Answer from the drawing. Dimensions are ordinates in mm from the lowest x, y and z of the part. Give positions to 0.01 mm unless a question says otherwise; leave off trailing zeros. Loops run counter-clockwise (first coordinate to the right, second up) from the corner with the lowest first, then second, coordinate; pieces in that order, holes last.
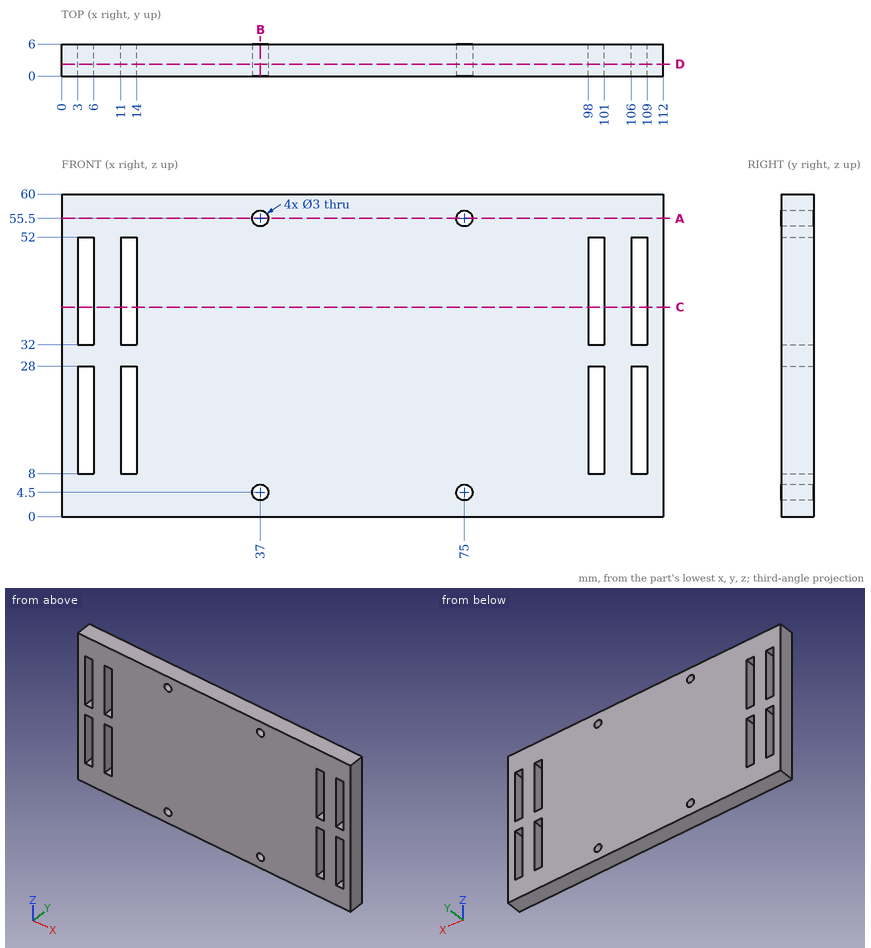
Item 1: Consider line 1 (X direction, y = 2.55, z = 4.5); line 2 (X direction, y = 5.7, z = 18); line 3 (Z direction, x = 75, y = 1.25). Determine where each line is inside the solid, lowest interval first.
Item 2: Find section B-B, the plane x = 37. Write down the section's boundary in (y, z).
Item 3: Find section C-C, the plane z = 39. Write down the section's boundary in (x, y), plus the area to 3 significant figures.
Item 4: Find section A-A, the plane z = 55.5. Write down the section's boundary in (x, y), plus the area to 3 significant figures.
Item 5: A flat-ended cylindrical pin translates along its axis: pin 1 Ø1.8 at (y, z) = (2.5, 18.5) entering from -X. Find the tip coordinate at first contact, or state that the pin passes through.
Item 6: Find section D-D, the plane y = 2.25. Give the number of separate pieces and of enclosed holes in the cut face, plus the area to 3 significant figures.
Ans:
1. line 1: x = 0 to 35.5, 38.5 to 73.5, 76.5 to 112
1. line 2: x = 0 to 3, 6 to 11, 14 to 98, 101 to 106, 109 to 112
1. line 3: z = 0 to 3, 6 to 54, 57 to 60
2. outline: (0, 0) - (6, 0) - (6, 3) - (0, 3) - close; (0, 6) - (6, 6) - (6, 54) - (0, 54) - close; (0, 57) - (6, 57) - (6, 60) - (0, 60) - close
3. outline: (0, 0) - (3, 0) - (3, 6) - (0, 6) - close; (6, 0) - (11, 0) - (11, 6) - (6, 6) - close; (14, 0) - (98, 0) - (98, 6) - (14, 6) - close; (101, 0) - (106, 0) - (106, 6) - (101, 6) - close; (109, 0) - (112, 0) - (112, 6) - (109, 6) - close
3. area: 600 mm2
4. outline: (0, 0) - (35.5, 0) - (35.5, 6) - (0, 6) - close; (38.5, 0) - (73.5, 0) - (73.5, 6) - (38.5, 6) - close; (76.5, 0) - (112, 0) - (112, 6) - (76.5, 6) - close
4. area: 636 mm2
5. pin 1: stops at x = 0
6. separate pieces: 1
6. enclosed holes: 12
6. area: 6,210 mm2
